The listing builds one solid part. Answer for the finished solid, in the listing's coordinates (mm). Face numbers are marked on the shaded views. A direction names the side the tool comes from. Coordinates: 2 decimals unless noted, no trailing zeros. Loops run counter-clockwise (first coordinate to the right, second up) from the corner with the lowest first, then second, coordinate; pieces in that order, holes last. Notation, with made-up numbers: (81, 15.5) -> (89, 15.5) arc R27 cw to (89, 50.5) -> close; hole circle Ø10 at (70.5, -26). An arc over 180 degrees is marked (long way). Answer in a Markdown table with one row per item.
Autodesk Inventor part; units mm, degrees
ref_plane "Work Plane1" through (-15.2152, -6.2652, -4.8) normal (0, 0, 1) x (1, 0, 0)
ref_plane "Work Plane2" through (-2.5323, -0.0859, -0.8) normal (0, 0, -1) x (0, 1, 0)
ref_plane "YZ Plane" through (0, 0, 0) normal (1, 0, 0) x (0, 1, 0)
sketch "Sketch1" plane through (0, 0, 0) normal (0, 0, 1) x (1, 0, 0)
  circle A0 centre (0, 8.95) radius 1.09
  arc A1 (1.662, 7.8375) -> (-0.0143, 6.9501) centre (0, 8.95) ccw
  arc A2 (1.8983, 9.5797) -> (-1.8983, 9.5797) centre (0, 8.95) ccw
  line L0 (3.6, 4.45) -> (3.6, -5.6116)
  arc A3 (-3.6, -5.6116) -> (3.6, -5.6116) centre (0, 8.95) ccw
  circle A4 centre (0, 8.95) radius 4.08
  circle A5 centre (0, 8.95) radius 15
  line L1 (2.5, -0.05) -> (2.5, 4.45)
  line L2 (2.5, 4.45) -> (3.6, 4.45)
  line L3 (3.6, 4.45) -> (3.6, -4.45)
  line L4 (3.6, -4.45) -> (-3.6, -4.45)
  line L5 (-3.6, -4.45) -> (-3.6, 4.45)
  line L6 (-3.6, 4.45) -> (-2.5, 4.45)
  line L7 (-2.5, 4.45) -> (-2.5, -0.05)
  line L8 (-3.6, -5.6116) -> (-3.6, 4.45)
  line L9 (-3.6, 4.45) -> (-1.8983, 9.5797)
  line L10 (3.6, 4.45) -> (1.8983, 9.5797)
  line L11 (-2.5, -0.05) -> (2.5, -0.05)
  point P0 (0, 0)
  point P1 (-1.8983, 9.5797)
extrude "Extrusion1" add sketch "Sketch1" along normal blind 2 contours L10 A4 L9 A1 | L10 L2 L1 L11 L7 L6 L9 A4 | L0 L4 L5 L6 L7 L11 L1 L2 | L0 A3 L8 L4 picked at (1.9915, 8.1578)
sketch "Sketch2" plane through (0, 0, 0) normal (0, 0, -1) x (-1, 0, 0)
  line L0 (-3.6, -4.45) -> (3.6, -4.45)
  line L1 (-3.6, 4.45) -> (-1.8983, 9.5797)
  line L2 (-3.6, -5.6116) -> (-3.6, 4.45)
  arc A0 (-3.6, -5.6116) -> (3.6, -5.6116) centre (0, 8.95) ccw
  line L3 (3.6, 4.45) -> (3.6, -5.6116)
  line L4 (1.8983, 9.5797) -> (3.6, 4.45)
  arc A1 (1.8983, 9.5797) -> (-1.8983, 9.5797) centre (0, 8.95) ccw
  circle A2 centre (0, 8.95) radius 1.09
  point P0 (0, 0)
ref_plane "Work Plane1" through (-15.2152, -6.2652, -4.8) normal (0, 0, 1) x (1, 0, 0)
extrude "Extrusion2" add sketch "Sketch2" along normal up to surface (4.8 mm away) contours L0 L3 A0 L2
sketch "Sketch3" plane through (-3.6, -4.45, 0) normal (0, 1, 0) x (1, 0, 0)
  circle A0 centre (3.6, 2.8) radius 1.6
  point P0 (3.6, 0)
extrude "Extrusion3" cut sketch "Sketch3" against normal blind 10
fillet "Fillet1" radius 1 6 edges at (2.7491, 7.0149, 2) (3.6, -0.5808, 2) (0, -6.05, 2) (-3.6, -0.5808, 2) (-2.7491, 7.0149, 2) (0, 10.95, 2)
sketch "Sketch4" plane through (0, 0, 0) normal (0, 0, -1) x (-1, 0, 0)
  point P0 (0, 0)
sketch "Sketch5" plane through (0, 0, 0) normal (0, 0, -1) x (-1, 0, 0)
  line L0 (-3.6, 4.45) -> (3.6, 4.45)
  arc A0 (0.0143, 6.9501) -> (-1.662, 7.8375) centre (0, 8.95) ccw
  circle A1 centre (0, 8.95) radius 1.09
  line L1 (-3.8923, -4.5783) -> (-11.4921, -4.6328)
  line L2 (-11.4921, -4.6328) -> (-11.5941, 9.5788)
  line L3 (-3.3887, 7.8251) -> (-11.5941, 9.5788)
  line L4 (-1.662, 7.8375) -> (-3.3887, 7.8251)
  arc A2 (0.0143, 6.9501) -> (-1.662, 7.8375) centre (0, 8.95) ccw
  line L5 (0.0143, 6.9501) -> (-1.9749, 6.9358)
  arc A3 (-1.9749, 6.9358) -> (-3.9605, 4.9215) centre (-1.9605, 4.9358) ccw
  line L6 (-3.9605, 4.9215) -> (-3.8923, -4.5783)
  line L7 (-10.8065, -2.6278) -> (-4.6067, -2.5833)
  line L8 (-4.6067, -2.5833) -> (-4.6246, -0.0834)
  line L9 (-4.6246, -0.0834) -> (-10.8244, -0.1279)
  line L10 (-10.8244, -0.1279) -> (-10.8065, -2.6278)
  line L11 (-3.6, 4.45) -> (-1.8983, 9.5797)
  line L12 (-3.6, 4.45) -> (-2.8435, 6.7304)
  line L13 (1.8983, 9.5797) -> (2.0348, 9.1681)
  line L14 (3.6, 4.45) -> (1.8983, 9.5797)
  arc A4 (0.0151, 6.8501) -> (-1.7451, 7.7818) centre (0, 8.95) ccw
  line L15 (0.0151, 6.8501) -> (-1.9742, 6.8358)
  arc A5 (-1.9742, 6.8358) -> (-3.8605, 4.9222) centre (-1.9605, 4.9358) ccw
  line L16 (-3.8605, 4.9222) -> (-3.7916, -4.6775)
  line L17 (-3.7916, -4.6775) -> (-11.5914, -4.7335)
  line L18 (-11.5914, -4.7335) -> (-11.695, 9.7026)
  line L19 (-11.695, 9.7026) -> (-3.3785, 7.9252)
  line L20 (-3.3785, 7.9252) -> (-1.6627, 7.9375)
  point P0 (0, 0)
  point P1 (2.0999, 8.972)
  point P2 (0.0151, 6.8501)
  point P3 (-2.8889, 6.5936)
  dimension "d7" = 0.1
  dimension "d8" = 0.1
ref_plane "Work Plane2" through (-2.5323, -0.0859, -0.8) normal (0, 0, -1) x (0, 1, 0)
extrude "Extrusion4" add sketch "Sketch5" along normal up to surface (0.8 mm away) contours L11 A5 L15 A4 L14 L0
properties part number "Tool Head Clamp"
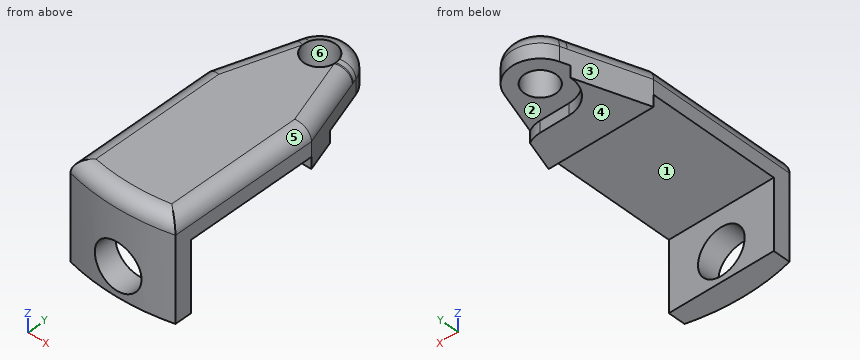
Item 1: A tool of negligible diameter and unlimited length cuts with its end or side. For the marked faces 1, 2 and 3, from which of +Z, -Z, +X, -X, +Y, -Y can it reach the whole face along a straight path? Write none if from no direction.
Findings below:
| item | result |
|---|---|
| face 1 | -Z, +X, -X |
| face 2 | -Z, +X, +Y |
| face 3 | +Z, -Z, -X, +Y |
Item 2: Find the intervals of material crossed by probe 1 along Z at (x, y) = (0, -4.75); probe 2 along Y at (x, z) = (0, 0.8); probe 3 along X at (y, z) = (-4.85, -2.8), in increasing order.
Findings below:
| item | result |
|---|---|
| probe 1 | z = -4.8 to -4.4, -1.2 to 2 |
| probe 2 | y = -6.05 to 7.86, 10.04 to 10.95 |
| probe 3 | x = -3.6 to -1.6, 1.6 to 3.6 |
Item 3: Determine the mould class of the marked faces 4, 5 and 6 for opening direction X: +X half, -X half, draft (parallel to the pull), parting line (faces both ways), or undercut.
Findings below:
| item | result |
|---|---|
| face 4 | draft |
| face 5 | +X half |
| face 6 | undercut |
Item 4: A cutting plane is placed at C-C, the plane z = -0.5. Determine the outline of the cut face in (x, y), plus the area to 3 significant figures.
Findings below:
| item | result |
|---|---|
| outline | (-3.6, -5.61) arc R15 ccw to (3.6, -5.61) -> (3.6, -4.45) -> (-3.6, -4.45) -> close; (-3.6, 4.45) -> (3.6, 4.45) -> (2.89, 6.59) arc R1.9 ccw to (1.97, 6.84) -> (-0.02, 6.85) arc R2.1 cw to (-2.1, 8.97) -> close |
| area | 27.4 mm2 |
Item 5: Flat-ended cylindrical pins translate along their axes: pin 1 Ø0.9 at (x, z) = (-1.5, -0.5) entering from -Y; pin 2 Ø2 at (x, y) = (0, 9) entering from -Z; pin 3 Ø2.5 at (x, y) = (0, 7.5) entering from -Z. Find the tip coordinate at first contact, or state that the pin passes through.
Findings below:
| item | result |
|---|---|
| pin 1 | stops at y = -6.01 |
| pin 2 | passes through |
| pin 3 | stops at z = -0.8 |
Item 6: A cutting plane is placed at A-A, the plane z = -2.8. Determine the outline of the cut face in (x, y).
Findings below:
| item | result |
|---|---|
| outline | (-3.6, -5.61) arc R15 ccw to (-1.6, -5.96) -> (-1.6, -4.45) -> (-3.6, -4.45) -> close; (1.6, -5.96) arc R15 ccw to (3.6, -5.61) -> (3.6, -4.45) -> (1.6, -4.45) -> close |
Item 7: A cutting plane is placed at B-B, the plane y = -4.25. Determine the outline of the cut face in (x, z), plus the area to 3 significant figures.
Findings below:
| item | result |
|---|---|
| outline | (-3.6, 0) -> (3.6, 0) -> (3.6, 1) arc R1 ccw to (2.6, 2) -> (-2.6, 2) arc R1 ccw to (-3.6, 1) -> close |
| area | 14.0 mm2 |
